```python
from build123d import *

# Parameters (mm, degrees)
SKETCH1_W           = 50.8
SKETCH1_H           = 152.4
BOSS_EXTRUDE1_DEPTH = 50.8
SHELL1_T            = -6.35
SKETCH4_R           = 14.075
CUT_EXTRUDE1_DEPTH  = 25


with BuildPart() as part:
    # Sketch1 → Boss-Extrude1 (new body)
    with BuildSketch(Plane(origin=(0, 0, 0), x_dir=(1, 0, 0), z_dir=(0, 1, 0))):
        with Locations((25.4, 76.2)):
            Rectangle(SKETCH1_W, SKETCH1_H)
    extrude(amount=BOSS_EXTRUDE1_DEPTH)

    # Shell1
    shell1_openings = [part.faces().sort_by_distance(p)[0] for p in [
        (0, 25.4, -76.2),
    ]]
    offset(amount=SHELL1_T, openings=shell1_openings, kind=Kind.INTERSECTION)

    # Sketch4 → Cut-Extrude1 (cut)
    with BuildSketch(Plane(origin=(50.8, 0, 0), x_dir=(0, 0, -1), z_dir=(1, 0, 0))):
        with Locations((113.988045791, 25.683455189)):
            Circle(SKETCH4_R)
    extrude(amount=-CUT_EXTRUDE1_DEPTH, mode=Mode.SUBTRACT)


solid = part.part
```
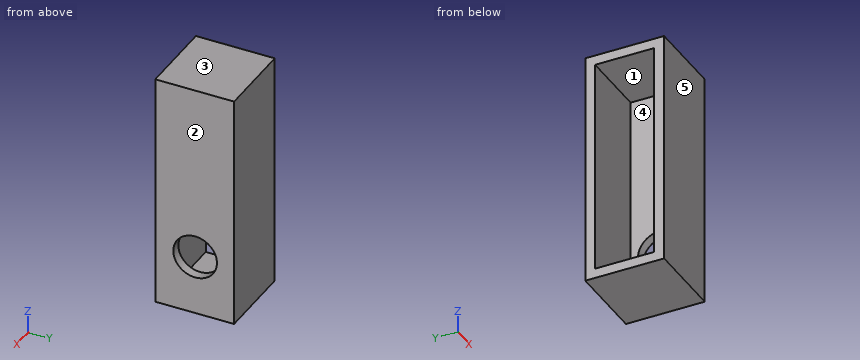
Here's how the part is built. I have some questions about the finished solid (model axes, mm). Face numbers are marked on the shaded views. A direction names the side the tool comes from. Coordinates: 2 decimals unless noted, no trailing zeros. Order: outer loops, then holes, each group sorted by start corner. A loop starts at its lowest first (then second) coordinate and runs counter-clockwise, first axis right, second up.
1) Imagine slicing it at B-B on x = 32. List the corners of the cut face in (y, z) for me.
2) Will these pins go through, and if not, where does the flat tip stop? pin 1 (19 mm diameter, centred on x = 11.5, y = 28.5, fed in from +Z); pin 2 (19 mm diameter, centred on y = 18, z = -97.5, fed in from -X); pin 3 (22.5 mm diameter, centred on y = 25.68, z = -113.99, fed in from -X).
3) Which directions (+Z, -Z, +X, -X, +Y, -Y) give clear straight access to the entire face, cutting with the end or side of a thin tool? Please do the marked faces 1 and 2.
4) Imagine slicing it at A-A on z = -111.5. List the corners of the cut face in (x, y) for me.
5) We'd pull the mould along Y, two halves only. Please class the marked faces 3, 4 and 5: +Y half, -Y half, draft (parallel to the pull), parting line (faces both ways), or undercut.
6) Imagine slicing it at C-C on y = 33. List the corners of the cut face in (x, z) for me.
7) Imagine slicing it at D-D on z = -140.5. List the corners of the cut face in (x, y) for me.
8) I need wall thicknesses on line 1 (Y direction, x = 35, z = -37.5); line 2 (Z direction, x = 29, y = 24). Which ranges of each line are inside material? Lowest first, please.
Response values:
1. outline: (0, -152.4) - (50.8, -152.4) - (50.8, 0) - (0, 0) - close; hole (6.35, -146.05) - (44.45, -146.05) - (44.45, -6.35) - (6.35, -6.35) - close
2. pin 1: stops at z = 0
2. pin 2: stops at x = 44.45
2. pin 3: passes through
3. face 1: -X
3. face 2: +Z, -Z, +X, +Y, -Y
4. outline: (0, 0) - (50.8, 0) - (50.8, 11.83) - (44.45, 11.83) - (44.45, 6.35) - (0, 6.35) - close; (0, 44.45) - (44.45, 44.45) - (44.45, 39.54) - (50.8, 39.54) - (50.8, 50.8) - (0, 50.8) - close
5. face 3: draft
5. face 4: undercut
5. face 5: -Y half
6. outline: (0, -152.4) - (50.8, -152.4) - (50.8, -126.01) - (44.45, -126.01) - (44.45, -146.05) - (0, -146.05) - close; (0, -6.35) - (44.45, -6.35) - (44.45, -101.96) - (50.8, -101.96) - (50.8, 0) - (0, 0) - close
7. outline: (0, 0) - (50.8, 0) - (50.8, 50.8) - (0, 50.8) - (0, 44.45) - (44.45, 44.45) - (44.45, 6.35) - (0, 6.35) - close
8. line 1: y = 0 to 6.35, 44.45 to 50.8
8. line 2: z = -152.4 to -146.05, -6.35 to 0
